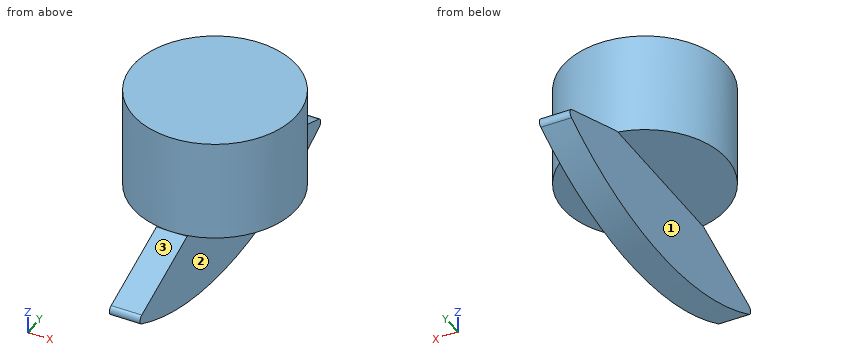
```python
from build123d import *

# Parameters (mm, degrees)
SKETCH_1_R           = 8
EXTRUDE_1_DEPTH      = 10
EXTRUDE_2_DEPTH      = 1.5
EXTRUDE_2_DEPTH_BACK = 1.5
FILLET_1_R           = 0.5


with BuildPart() as part:
    # Sketch 1 → Extrude 1 (new body)
    with BuildSketch(Plane.XY):
        Circle(SKETCH_1_R)
    extrude(amount=EXTRUDE_1_DEPTH)

    # Sketch 2 → Extrude 2 (add, two sides)
    with BuildSketch(Plane(origin=(0, 0, 0), x_dir=(0, 0, -1), z_dir=(1, 0, 0))) as extrude_2_sk:
        with BuildLine():
            Line((0, -8), (0, 8))
            Line((0, 8), (3.420201433, 17.396926208))
            ThreePointArc((3.420201433, 17.396926208), (8, 0), (3.420201433, -17.396926208))
            Line((3.420201433, -17.396926208), (0, -8))
        make_face()
    extrude(amount=EXTRUDE_2_DEPTH)
    extrude(extrude_2_sk.sketch, amount=-EXTRUDE_2_DEPTH_BACK)

    # Fillet 1
    fillet_1_edges = [part.edges().sort_by_distance(p)[0] for p in [
        (0, 17.396926208, -3.420201433),
        (0, -17.396926208, -3.420201433),
    ]]
    fillet(fillet_1_edges, radius=FILLET_1_R)


solid = part.part
```
Read the model definition and answer for the solid it produces. Units are mm, in the model's axes. Face numbers are marked on the shaded views. A direction names the side the tool comes from. Give positions to 0.01 mm unless a question says otherwise; leave off trailing zeros. Order: outer loops, then holes, each group sorted by start corner. A loop starts at its lowest first (then second) coordinate and runs counter-clockwise, first axis right, second up.
(1) Find section D-D (x = -4.25). Give the vertices of the cut face in (y, z).
(2) For the marked faces 1, 2 and 3, determine the directions among +Z, -Z, +X, -X, +Y, -Y from which every point of the face is accessible in a straight line to the end or side of a thin tool.
(3) Straight lines are drawn through the part: L1, parallel to Z at x = -4.5, y = -1; L2, parallel to X at y = -12, z = -2.5; L3, parallel to Y at x = 0.75, z = 6.25. For each, find the intervals that lie inside material, in ascending order.
(4) Find section C-C (z = 7). Give the vertices of the cut face in (x, y), plus the area to 3 significant figures.
(5) Given pin 1 (3.5 mm diameter, centred on x = 6, y = 4, fed in from -Z); pin 2 (1 mm diameter, centred on x = 1, z = 2, fed in from -Y); pin 3 (6.5 mm diameter, centred on y = 7.5, z = -5, fed in from +X), each flat-ended and moving along its own axis, determine where each tip first touches the part or whether it passes through.
(6) Find section A-A (y = -6). Give the vertices of the cut face in (x, z), plus the area to 3 significant figures.
Result sheet:
1. outline: (-6.78, 0) - (6.78, 0) - (6.78, 10) - (-6.78, 10) - close
2. face 1: -Z, -X, +Y, -Y
2. face 2: -Z, +X, +Y, -Y
2. face 3: +Z, +X, -X, -Y
3. L1: z = 0 to 10
3. L2: x = -1.5 to 1.5
3. L3: y = -7.96 to 7.96
4. outline: circle Ø16 at (0, 0)
4. area: 201 mm2
5. pin 1: stops at z = 0
5. pin 2: stops at y = -7.98
5. pin 3: stops at x = 1.5
6. outline: (-5.29, 0) - (-1.5, 0) - (-1.5, -7.49) - (1.5, -7.49) - (1.5, 0) - (5.29, 0) - (5.29, 10) - (-5.29, 10) - close
6. area: 128 mm2
